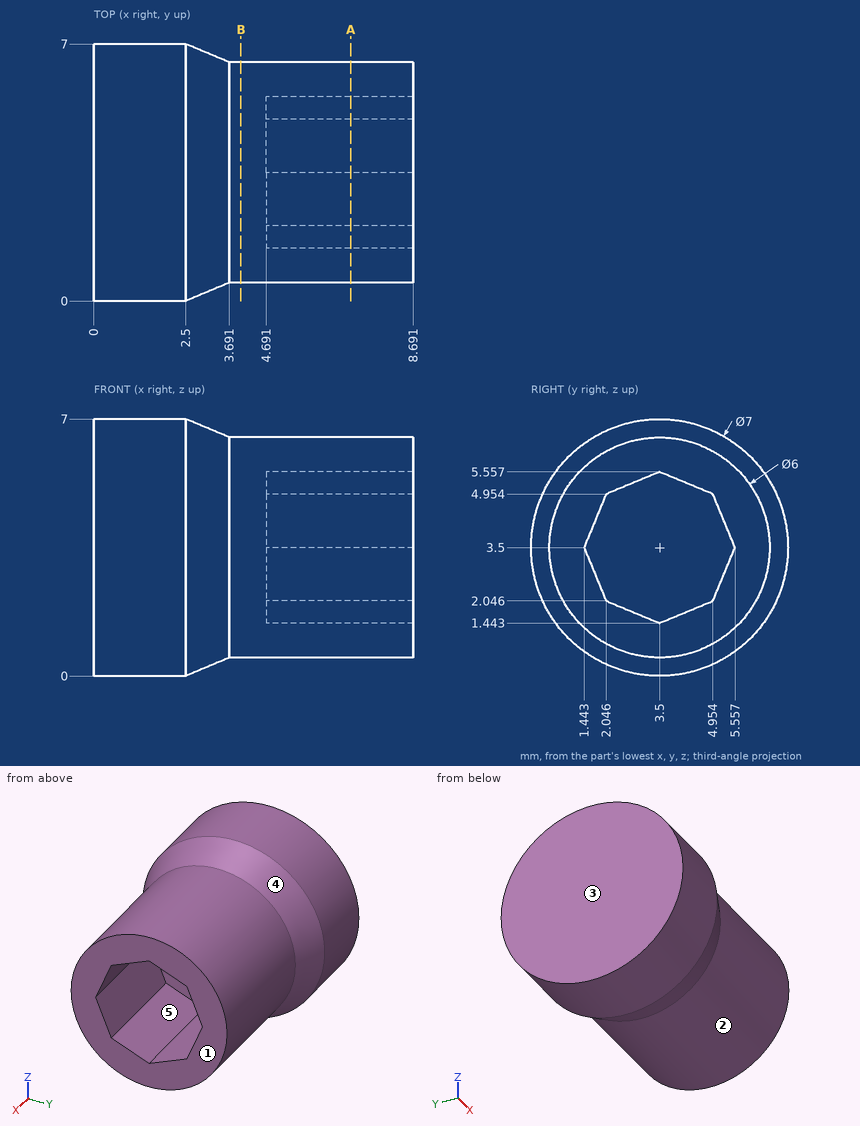
The drawing under review shows one solid part. Ordinate dimensions are in mm from its lowest x, y, z. A direction names the side the tool comes from. Round coordinates to 2 decimals unless told otherwise and drop trailing zeros. Loops run counter-clockwise (first coordinate to the right, second up) from the corner with the lowest first, then second, coordinate; pieces in that order, holes last. Notation, with made-up numbers: (6.25, 32) - (16.25, 32) arc R27 ccw to (16.25, 60) - close; hole circle Ø11 at (84, -1.75). An arc over 180 degrees is marked (long way). One line per item, written item: value. Start each with the question number.
1) Insertion check: pin 1 Ø1 at (x, z) = (5.5, 3) entering from -Y; pin 2 Ø4 at (x, z) = (4.5, 5.5) entering from -Y. Each pin has a flat end and moves straight along its axis. Give the tip position at first contact, or say it passes through.
2) Consider section A-A on x = 7. Give the boundary of the cut face in (y, z) (1 decimal).
3) For the marked faces 1 and 2, list the 3-axis set-ups (+Z, -Z, +X, -X, +Y, -Y) from which the entire face can be reached by the end or side of a thin tool; tool diameter is ignored.
4) Draft analysis for pull direction Y (two halves, no side actions). For the marked faces 3, 4 and 5, state which applies: +Y half, -Y half, draft (parallel to the pull), parting line (faces both ways), or undercut.
5) To check wall thickness, follow L1, parallel to Y at x = 8.25, z = 1.75 (1 decimal); L2, parallel to X at y = 2.25, z = 2.75; L3, parallel to Y at x = 6, z = 2.5. State the ranges of each line that lie inside material, in increasing order. Write a range as from..to.
6) Consider section B-B on x = 4. Give the boundary of the cut face in (y, z), then the cut area to 3 significant figures.
Reported:
1. pin 1: stops at y = 0.5
1. pin 2: stops at y = 0.26
2. outline: circle Ø6 at (3.5, 3.5); hole (1.4, 3.5) - (2, 2) - (3.5, 1.4) - (5, 2) - (5.6, 3.5) - (5, 5) - (3.5, 5.6) - (2, 5) - close
3. face 1: +Z, -Z, +X, +Y, -Y
3. face 2: +X
4. face 3: draft
4. face 4: parting line
4. face 5: undercut
5. L1: y = 1.1..2.8, 4.2..5.9
5. L2: x = 0..4.69
5. L3: y = 0.67..1.86, 5.14..6.33
6. outline: circle Ø6 at (3.5, 3.5)
6. area: 28.3 mm^2
